For this review, use the dimensioned drawing (mm, ordinates from the lowest corner) and the shaded views. A direction names the side the tool comes from. Coordinates: 2 decimals unless noted, no trailing zeros. Order: outer loops, then holes, each group sorted by start corner. A loop starts at its lowest first (then second) coordinate and runs counter-clockwise, first axis right, second up. Notation, with made-up numbers: M 71,-39 L 79,-39 A16 cw 79,-21 Z; hole C 74.25,77.5 d9. An arc over 180 degrees is marked long. One line per item, written item: value.
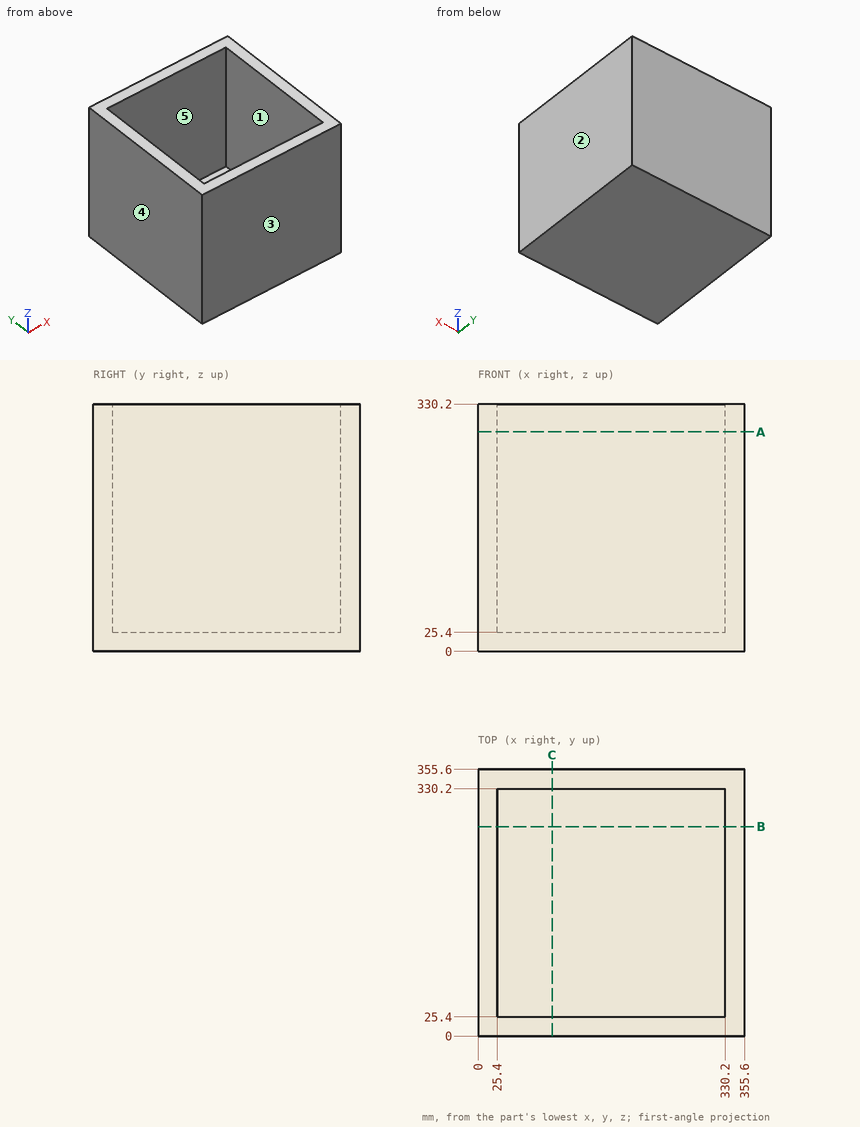
(1) Insertion check: pin 1 Ø8 at (x, y) = (244.5, 304.5) entering from +Z. The pin has a flat end and moves straight along its axis. Give the tip position at first contact, or say it passes through.
Geometry results:
pin 1: stops at z = 25.4
(2) Mouldability with a two-part tool opening along Y and no side actions: class the marked faces 1, 2 and 3 as +Y half, -Y half, draft (parallel to the pull), parting line (faces both ways), or undercut.
Geometry results:
face 1: undercut
face 2: draft
face 3: -Y half
(3) For L1, parallel to X at y = 182.5, z = 263; L2, parallel to Z at x = 259, y = 235.5, list the stretches that pass through material, from the lowest coordinate up.
Geometry results:
L1: x = 0 to 25.4, 330.2 to 355.6
L2: z = 0 to 25.4
(4) We need section B-B, the plane y = 279.5. State the section outline as (x, z) points.
Geometry results:
outline: M 0,0 L 355.6,0 L 355.6,330.2 L 330.2,330.2 L 330.2,25.4 L 25.4,25.4 L 25.4,330.2 L 0,330.2 Z
(5) We need section A-A, the plane z = 293. State the section outline as (x, y) points, plus the area to 3 significant figures.
Geometry results:
outline: M 0,0 L 355.6,0 L 355.6,355.6 L 0,355.6 Z; hole M 25.4,25.4 L 330.2,25.4 L 330.2,330.2 L 25.4,330.2 Z
area: 33,500 mm2
(6) Tool access review of the marked faces 4 and 5: name each direction out of +Z, -Z, +X, -X, +Y, -Y from which nothing blocks a thin tool from reaching the whole face with its end or side.
Geometry results:
face 4: +Z, -Z, -X, +Y, -Y
face 5: +Z
